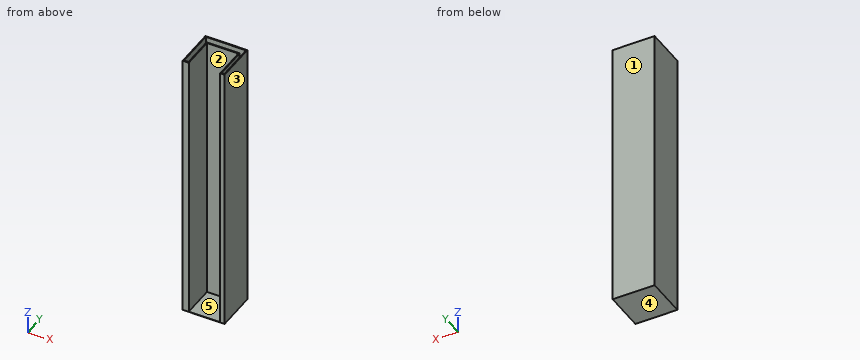
from build123d import *

# Parameters (mm, degrees)
F0_W        = 120.9424138069
F0_H        = 117.7590936422
F1_DEPTH    = 1
F4_DEPTH    = 25.4
F5_DEPTH    = 762
F6_T        = 2.54
F6_T3_DEPTH = 792.48
F6_T5_DEPTH = 99.200644033
F6_T7_DEPTH = 95.3667019176


# Not quite as in the source:
# - a shell that OpenCascade refuses in one call is made with other operations: the cavity is built on its own and cut out


with BuildPart() as f1:
    # F0 (on Top) → F1 (new body)
    with BuildSketch(Plane.XY):
        Rectangle(F0_W, F0_H)
    extrude(amount=F1_DEPTH)

    # F3 (on face) → F4 (join)
    with BuildSketch(Plane.XY.offset(1)):
        Polygon((-60.4712069035, 58.8795468211), (-60.4712069035, -58.8795468211), (-42.7266806364, -58.8795468211), (-42.7266806364, 35.2410972118), (47.5600212812, 35.2410972118), (47.5600212812, -58.8795468211), (60.4712069035, -58.8795468211), (60.4712069035, 58.8795468211), align=None)
    extrude(amount=F4_DEPTH)

    # F5 (add): a face of the model
    f5_faces = [f1.faces().sort_by_distance(p)[0] for p in [
        (-58.7831822711, 0, 26.4),
    ]]
    extrude(f5_faces, amount=F5_DEPTH)

    # F6: shell of thickness 2.54, made by hand


with BuildPart() as f6_core1:
    # F6_t2: copy of F1
    add(f1.part)

    # the walls: a layer under each face that stays
    f6_faces = [f6_core1.faces().sort_by_distance(p)[0] for p in [
        (0, 58.8795468211, 394.2),
        (0, 0, 0),
        (-51.8324630601, -58.8795468211, 732.0857142857),
        (47.5600212812, -11.8192248046, 394.7),
        (2.4166703224, 35.2410972118, 394.7),
        (2.4166703224, -11.8192248046, 1),
        (-42.7266806364, -11.8192248046, 394.7),
        (-60.4712069035, 0, 394.2),
        (60.4712069035, 0, 394.2),
    ]]
    thicken(f6_faces, amount=-F6_T, mode=Mode.SUBTRACT)

    # F6_s4 → F6_t3 (cut)
    with BuildSketch(Plane.XY.offset(-1.54)):
        Polygon((47.5346212812, 35.2156972118), (50.1000212812, 35.2410972118), (50.1000212812, 37.7810972118), (47.5600212812, 37.7810972118), align=None)
        Polygon((-42.7012806364, 35.2156972118), (-42.7266806364, 37.7810972118), (-45.2666806364, 37.7810972118), (-45.2666806364, 35.2410972118), align=None)
    extrude(amount=F6_T3_DEPTH, mode=Mode.SUBTRACT)

    # F6_s6 → F6_t5 (cut)
    with BuildSketch(Plane.XZ.offset(-37.7810972118)):
        Polygon((47.5346212812, 1.0254), (50.1000212812, 1), (50.1000212812, -1.54), (47.5600212812, -1.54), align=None)
        Polygon((-42.7012806364, 1.0254), (-42.7266806364, -1.54), (-45.2666806364, -1.54), (-45.2666806364, 1), align=None)
    extrude(amount=F6_T5_DEPTH, mode=Mode.SUBTRACT)

    # F6_s8 → F6_t7 (cut)
    with BuildSketch(Plane.YZ.offset(-45.2666806364)):
        Polygon((35.2156972118, 1.0254), (37.7810972118, 1), (37.7810972118, -1.54), (35.2410972118, -1.54), align=None)
    extrude(amount=F6_T7_DEPTH, mode=Mode.SUBTRACT)


with BuildPart() as f1_1:
    add(f1.part)

    # what is left inside the walls is the cavity
    f6_cavity = [f6_core1.part.solids().sort_by_distance(p)[0] for p in [
        (0, 56.314147, 526.446667),
    ]]
    add(f6_cavity, mode=Mode.SUBTRACT)


solid = f1_1.part
Build history of the part. All positions in model axes, mm. Face numbers are marked on the shaded views. A direction names the side the tool comes from. Give positions to 0.01 mm unless a question says otherwise; leave off trailing zeros. Write each loop counter-clockwise with the first axis right and the second up, starting at its lowest first coordinate (ties: lowest second). Pieces come first, ordered by that corner, then holes. Notation, with made-up numbers: (-32, -8.5) - (-19, -8.5) arc R34 ccw to (-19, 28.5) - close; hole circle Ø3 at (-7.5, 72). An arc over 180 degrees is marked (long way). Use one line per item in the form item = value. Start each with the question number.
1. Two-plate mould, pull along X, no slides. Class the marked faces 1, 2 and 3: released by +X, released by -X, zero draft, split by the parting line, or undercut.
2. Band-saw the part on A-A on z = 147. Write the cut outline in (x, y).
3. Drop flat-ended pins along their axis: pin 1 Ø10 at (x, y) = (21.5, -37.5) entering from +Z; pin 2 Ø2 at (x, z) = (-38.5, 378.5) entering from -Y. Give the stop position or say it passes through.
4. 3-axis set-ups, long thin cutter, end or side, ignore diameter. For the marked faces 4 and 5: which of +Z, -Z, +X, -X, +Y, -Y reach the whole face in a straight line?
5. Band-saw the part on B-B on y = -11. Write the cut outline in (x, z), plus the area to 3 significant figures.
6. Band-saw the part on C-C on x = 36.5. Write the cut outline in (y, z).
7. Probe line 1 (X direction, y = -33.5, z = 563); line 2 (Y direction, x = 9, z = 395); line 3 (Y direction, x = -44, z = 147). List the from-to ranges inside material, lowest first. Write a range as [from, to].
Conclusion:
q1.face_1 = zero draft
q1.face_2 = undercut
q1.face_3 = released by +X
q2.outline = (-60.47, -58.88) - (-42.73, -58.88) - (-42.73, 35.24) - (47.56, 35.24) - (47.56, -58.88) - (60.47, -58.88) - (60.47, 58.88) - (-60.47, 58.88) - close; hole (-57.93, -56.34) - (-45.27, -56.34) - (-45.27, 37.78) - (50.1, 37.78) - (50.1, -56.34) - (57.93, -56.34) - (57.93, 56.34) - (-57.93, 56.34) - close
q3.pin_1 = 1
q3.pin_2 = 35.24
q4.face_4 = -Z, +X, -X, +Y, -Y
q4.face_5 = +Z, -Y
q5.outline = (-60.47, 0) - (60.47, 0) - (60.47, 788.4) - (57.93, 788.4) - (57.93, 2.54) - (50.1, 2.54) - (50.1, 788.4) - (47.56, 788.4) - (47.56, 1) - (-42.73, 1) - (-42.73, 788.4) - (-45.27, 788.4) - (-45.27, 2.54) - (-57.93, 2.54) - (-57.93, 788.4) - (-60.47, 788.4) - close
q5.area = 8,150 mm²
q6.outline = (-58.88, 0) - (58.88, 0) - (58.88, 788.4) - (56.34, 788.4) - (56.34, 2.54) - (37.78, 2.54) - (37.78, 788.4) - (35.24, 788.4) - (35.24, 1) - (-58.88, 1) - close
q7.line_1 = [-60.47, -57.93], [-45.27, -42.73], [47.56, 50.1], [57.93, 60.47]
q7.line_2 = [35.24, 37.78], [56.34, 58.88]
q7.line_3 = [-58.88, 37.78], [56.34, 58.88]
